```python
from build123d import *

# Parameters (mm, degrees)
SKETCH1_R           = 8
BOSS_EXTRUDE1_DEPTH = 5
BOSS_EXTRUDE2_START = 5
SKETCH1_3_R         = 105
BOSS_EXTRUDE2_DEPTH = 50
BOSS_EXTRUDE3_START = 55
SKETCH1_4_R         = 8
SKETCH1_4_R_2       = 105
BOSS_EXTRUDE3_DEPTH = 10
SKETCH2_R           = 15


with BuildPart() as part:
    # Sketch1 → Boss-Extrude1 (new body, symmetric)
    with BuildSketch(Plane.XY):
        with BuildLine():
            Line((-25, 240.330386365), (-25, 101.980390272))
            ThreePointArc((-25, 101.980390272), (-64.807406984, -82.613558209), (105, 0))
            Line((105, 0), (105, 290))
            Line((105, 290), (42.740477075, 290))
            Line((42.740477075, 290), (42.740477075, 240.330386365))
            Line((42.740477075, 240.330386365), (-25, 240.330386365))
        make_face()
        with Locations((0, 220)):
            Circle(SKETCH1_R, mode=Mode.SUBTRACT)
    extrude(amount=BOSS_EXTRUDE1_DEPTH, both=True)

    # Sketch1<3> → Boss-Extrude2 (add)
    with BuildSketch(Plane.XY.offset(BOSS_EXTRUDE2_START)):
        Circle(SKETCH1_3_R)
    extrude(amount=BOSS_EXTRUDE2_DEPTH)

    # Sketch1<4> → Boss-Extrude3 (add)
    with BuildSketch(Plane.XY.offset(BOSS_EXTRUDE3_START)):
        with BuildLine():
            ThreePointArc((-25, 101.980390272), (64.807406984, 82.613558209), (105, 0))
            Line((105, 0), (105, 290))
            Line((105, 290), (42.740477075, 290))
            Line((42.740477075, 290), (42.740477075, 240.330386365))
            Line((42.740477075, 240.330386365), (-25, 240.330386365))
            Line((-25, 240.330386365), (-25, 101.980390272))
        make_face()
        with Locations((0, 220)):
            Circle(SKETCH1_4_R, mode=Mode.SUBTRACT)
        Circle(SKETCH1_4_R_2)
    extrude(amount=BOSS_EXTRUDE3_DEPTH)


with BuildPart() as body_2:
    # Sketch2 → Revolve1 (revolve)
    with BuildSketch(Plane(origin=(0, 0, 0), x_dir=(0, 0, -1), z_dir=(1, 0, 0))):
        with Locations((-30, 105)):
            Circle(SKETCH2_R)
    revolve(axis=Axis((0, 0, 45), (0, 0, -1)))


with BuildPart() as part_1:
    add(part.part)

    # Combine1: cut body 2
    add(body_2.part, mode=Mode.SUBTRACT)


solid = part_1.part
```
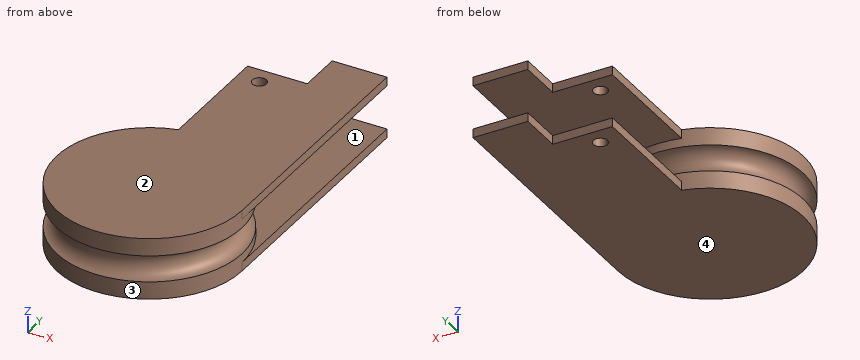
Input: part model. Units: mm. Frame: model coordinates. Face numbers are marked on the shaded views. Give positions to 0.01 mm unless a question says otherwise; leave off trailing zeros. Order: outer loops, then holes, each group sorted by start corner. A loop starts at its lowest first (then second) coordinate and runs counter-clockwise, first axis right, second up. Notation, with made-up numbers: M 42,-14 L 88,-14 A35 ccw 88,25 Z; hole C 86,61.5 d8. An arc over 180 degrees is marked long. Return JSON: item names as keys, results as strings.
1) Section query A-A on y = 195.5. Output: boundary loops of the cut face in (x, z), and give its area (3 significant figures).
Taken from the geometry:
{"outline": "M -25,-5 L 105,-5 L 105,5 L -25,5 Z; M -25,55 L 105,55 L 105,65 L -25,65 Z", "area": "2,600 mm2"}
2) Line query: L1, parallel to Z at x = 92.5, y = 107.5; L2, parallel to Y at x = 0, z = 2; L3, parallel to X at y = 133.5, z = 4. Output: solid intervals per line, ascending. Write a range as [from, to].
Taken from the geometry:
{"L1": "z = [-5, 5], [55, 65]", "L2": "y = [-105, 212], [228, 240.33]", "L3": "x = [-25, 105]"}
3) Section query C-C on z = 23. Output: boundary loops of the cut face in (x, y), and give its area (3 significant figures).
Taken from the geometry:
{"outline": "C 0,0 d183.47", "area": "26,400 mm2"}
4) Mould query, pull axis Z, two halves, no side actions, for the marked faces 1, 2, 3 and 4. Classes: released by +Z, released by -Z, zero draft, split by the parting line, or undercut.
Taken from the geometry:
{"face 1": "undercut", "face 2": "released by +Z", "face 3": "undercut", "face 4": "released by -Z"}
5) Contact query for flat-ended pins moving along their axis: pin 1 (13 mm diameter, centred on x = 0, y = 220, fed in from -Z); pin 2 (11 mm diameter, centred on x = 15.5, z = 60, fed in from +Y); pin 3 (1 mm diameter, centred on y = -50.5, z = 57.5, fed in from +X); pin 4 (11 mm diameter, centred on y = 274.5, z = 62.5, fed in from -X). Output: stop coordinate, or through.
Taken from the geometry:
{"pin 1": "passes through", "pin 2": "stops at y = 240.33", "pin 3": "stops at x = 92.33", "pin 4": "stops at x = 42.74"}
6) Section query B-B on x = 0. Output: boundary loops of the cut face in (y, z).
Taken from the geometry:
{"outline": "M -105,-5 L 212,-5 L 212,5 L 105,5 L 105,15 A15 cw 105,45 L 105,55 L 212,55 L 212,65 L -105,65 L -105,45 A15 cw -105,15 Z; M 228,-5 L 240.33,-5 L 240.33,5 L 228,5 Z; M 228,55 L 240.33,55 L 240.33,65 L 228,65 Z"}
